from build123d import *

# Parameters (mm, degrees)
BOSS_EXTRUDE1_DEPTH = 35
SKETCH3_W           = 3
SKETCH3_H           = 97.69244928
EXTRUDE_THIN1_DEPTH = 20


with BuildPart() as part:
    # Sketch1 → Boss-Extrude1 (new, symmetric)
    with BuildSketch(Plane.XY):
        Polygon((-26.646058096, 42.308244917), (26.646058096, -42.308244917), (45.155915247, -42.308244917), (45.155915247, -39.259184306), (27.963657577, -39.259184306), (-23.904623451, 43.526660315), align=None)
    extrude(amount=BOSS_EXTRUDE1_DEPTH, both=True)

    # Sketch3 → Extrude-Thin1 (add)
    with BuildSketch(Plane(origin=(2.417426631, 1.514603909, 0), x_dir=(0, 0, -1), z_dir=(0.8474129293595072, 0.5309343906306494, 0))):
        with Locations((-35.395786922, 0.730616768)):
            Rectangle(SKETCH3_W, SKETCH3_H)
        with Locations((31.987403947, 0.730616768)):
            Rectangle(SKETCH3_W, SKETCH3_H)
    extrude(amount=EXTRUDE_THIN1_DEPTH)


solid = part.part
The model under review builds one solid part; all positions refer to its coordinate system, in mm. A direction names the side the tool comes from. Round coordinates to 2 decimals unless told otherwise and drop trailing zeros. Order: outer loops, then holes, each group sorted by start corner. A loop starts at its lowest first (then second) coordinate and runs counter-clockwise, first axis right, second up. Notation, with made-up numbers: (-40, 63) -> (-4, 63) arc R10 cw to (-4, 78) -> close; hole circle Ø10 at (19.25, 18). An arc over 180 degrees is marked (long way). Return JSON: item names as keys, results as strings.
1. Take a section at C-C (y = 45). Write out the cut boundary in (x, z).
Answer block:
{"outline": "(-21.55, -33.49) -> (-1.23, -33.49) -> (-1.23, -30.49) -> (-21.55, -30.49) -> close; (-21.55, 33.9) -> (-1.23, 33.9) -> (-1.23, 36.9) -> (-21.55, 36.9) -> close"}
2. Take a section at A-A (x = 32.5). Write out the cut boundary in (y, z), then the cut area to 3 significant figures.
Answer block:
{"outline": "(-42.31, -35) -> (-39.26, -35) -> (-39.26, 35) -> (-42.31, 35) -> close; (-36.42, -33.49) -> (-8.83, -33.49) -> (-8.83, -30.49) -> (-36.42, -30.49) -> close; (-36.42, 33.9) -> (-8.83, 33.9) -> (-8.83, 36.9) -> (-36.42, 36.9) -> close", "area": "379 mm²"}
3. Take a section at D-D (y = 14). Write out the cut boundary in (x, z).
Answer block:
{"outline": "(-8.82, -35) -> (-5.41, -35) -> (-5.41, -33.49) -> (18.2, -33.49) -> (18.2, -30.49) -> (-5.41, -30.49) -> (-5.41, 33.9) -> (18.2, 33.9) -> (18.2, 36.9) -> (-5.41, 36.9) -> (-5.41, 35) -> (-8.82, 35) -> close"}
4. For faces 4 (the face through (2.393, 1.554, -34.233)), 5 (the face through (11, 7, 33.896)), 6 (the face through (-0.37, 0.59, 0.49)), 7 (the face through (36.319, -34.024, -31.966)), 8 (the face through (6, -6, 35)), list the 3-axis set-ups (+Z, -Z, +X, -X, +Y, -Y) from which the entire face can be reached by the end or side of a thin tool; tool diameter is ignored.
Answer block:
{"face 4": "-Z, +X, +Y", "face 5": "+X, +Y", "face 6": "+Z, -Z, -X, -Y", "face 7": "+Z, -Z, +X", "face 8": "+Z, -X, -Y"}
5. The part is to be moulded in two halves that separate along Y. For faces 1 (the face through (36.319, -34.024, 35.417)), 2 (the face through (18.615, 13.332, 35.417)), 3 (the face through (11, 7, -33.487)), say which applies: +Y half, -Y half, draft (parallel to the pull), parting line (faces both ways), or undercut.
Answer block:
{"face 1": "undercut", "face 2": "+Y half", "face 3": "draft"}
6. Insertion check: P1, Ø1.5, axis at y = -18.5, z = 9.5, coming from the +X side; P2, Ø1, axis at x = 7.5, z = 28, coming from the +Y side; P3, Ø1.5, axis at x = 2, z = 1.5, coming from the -Y side. Each pin has a flat end and moves straight along its axis. Give the tip position at first contact, or say it passes through.
Answer block:
{"P1": "stops at x = 15.43", "P2": "stops at y = -5.8", "P3": "stops at y = -4.37"}
7. Take a section at B-B (z = -13). Write out the cut boundary in (x, y).
Answer block:
{"outline": "(-26.65, 42.31) -> (26.65, -42.31) -> (45.16, -42.31) -> (45.16, -39.26) -> (27.96, -39.26) -> (-23.9, 43.53) -> close"}
8. For L1, parallel to Z at x = 17, y = 14; L2, parallel to Y at x = 30, z = 20; L3, parallel to Z at x = 1, y = -1, list the stretches that pass through material, from the lowest coordinate up. Write a range as [from, to].
Answer block:
{"L1": "z = [-33.49, -30.49], [33.9, 36.9]", "L2": "y = [-42.31, -39.26]", "L3": "z = [-35, 35]"}
